```python
from build123d import *

# Parameters (mm, degrees)
F0_R     = 2.38125
F1_DEPTH = 2.54
F2_R     = 40.005
F2_R_2   = 28.575
F2_R_3   = 2.38125
F3_DEPTH = 2.5410001


with BuildPart() as f1:
    # F0 (on Front) → F1 (new body)
    with BuildSketch(Plane.XZ):
        with BuildLine():
            ThreePointArc((6.3499999233, -24.9008008357), (-1.0762466814, -6.9535395158), (-19.0125346344, 0.4991715332))
            ThreePointArc((-19.0125346344, 0.4991715332), (-154.4493523287, -0.8097271588), (-289.8234049708, -5.1353108434))
            add(Edge.make_bspline(
                [(-289.8234049708, -5.1353108434), (-514.6487503932, -20.2006873557), (-514.3499970436, -90.5002)],
                knots=[4.9283667006, 4.9283667006, 4.9283667006, 6.2844832596, 6.2844832596, 6.2844832596], degree=2, weights=[1, 0.7787921925, 1]))
            Line((-514.3499970436, -90.5002), (-514.3499970436, -249.2502))
            ThreePointArc((-514.3499970436, -249.2502), (-506.9105092857, -267.2107122421), (-488.9499970436, -274.6502))
            Line((-488.9499970436, -274.6502), (-373.0752, -274.6502))
            ThreePointArc((-373.0752, -274.6502), (-337.1541755157, -259.7712244843), (-322.2752, -223.8502))
            Line((-322.2752, -223.8502), (-322.2752, -211.0369156084))
            ThreePointArc((-322.2752, -211.0369156084), (-303.2252, -191.9869156084), (-284.1752, -211.0369156084))
            Line((-284.1752, -211.0369156084), (-284.1752, -223.7369156084))
            ThreePointArc((-284.1752, -223.7369156084), (-269.2962244843, -259.6579400927), (-233.3752, -274.5369156084))
            Line((-233.3752, -274.5369156084), (-19.0500000767, -274.5369156084))
            ThreePointArc((-19.0500000767, -274.5369156084), (-1.0894878346, -267.0974278505), (6.3499999233, -249.1369156084))
            Line((6.3499999233, -249.1369156084), (6.3499999233, -24.9008008357))
        make_face()
        with Locations((-412.75, -261.9502)):
            Circle(F0_R, mode=Mode.SUBTRACT)
        with Locations((-180.975, -261.9502)):
            Circle(F0_R, mode=Mode.SUBTRACT)
        with Locations((-34.925, -261.9502)):
            Circle(F0_R, mode=Mode.SUBTRACT)
        with BuildLine():
            ThreePointArc((-177.8000000767, -147.5369156084), (-175.9401281373, -143.0467875478), (-171.4500000767, -141.1869156084))
            Line((-171.4500000767, -141.1869156084), (-25.4000000767, -141.1869156084))
            ThreePointArc((-25.4000000767, -141.1869156084), (-20.9098720162, -143.0467875478), (-19.0500000767, -147.5369156084))
            Line((-19.0500000767, -147.5369156084), (-19.0500000767, -242.7869156084))
            ThreePointArc((-19.0500000767, -242.7869156084), (-20.9098720162, -247.2770436689), (-25.4000000767, -249.1369156084))
            Line((-25.4000000767, -249.1369156084), (-171.4500000767, -249.1369156084))
            ThreePointArc((-171.4500000767, -249.1369156084), (-175.9401281373, -247.2770436689), (-177.8000000767, -242.7869156084))
            Line((-177.8000000767, -242.7869156084), (-177.8000000767, -203.9237609675))
            ThreePointArc((-177.8000000767, -203.9237609675), (-180.3400000767, -196.9399156084), (-177.8000000767, -189.9560702493))
            Line((-177.8000000767, -189.9560702493), (-177.8000000767, -147.5369156084))
        make_face(mode=Mode.SUBTRACT)
        with Locations((-438.15, -46.0502)):
            Circle(F0_R, mode=Mode.SUBTRACT)
        with Locations((-228.6, -14.1869156084)):
            Circle(F0_R, mode=Mode.SUBTRACT)
        with Locations((-19.05, -11.1252)):
            Circle(F0_R, mode=Mode.SUBTRACT)
    extrude(amount=F1_DEPTH)

    # F2 (on face) → F3 (cut, through all)
    with BuildSketch(Plane.XZ.offset(2.54)):
        with Locations((-50.8, -93.5619156084)):
            Circle(F2_R)
        with Locations((-139.7, -93.5619156084)):
            Circle(F2_R)
        with Locations((-228.6, -93.5619156084)):
            Circle(F2_R)
        with Locations((-304.8, -118.9619156084)):
            Circle(F2_R_2)
        with Locations((-19.05, -125.3119156084)):
            Circle(F2_R_3)
        with Locations((-82.5499999959, -125.3119156124)):
            Circle(F2_R_3)
        with Locations((-82.5500000081, -61.8119156165)):
            Circle(F2_R_3)
        with Locations((-19.0500000122, -61.8119155962)):
            Circle(F2_R_3)
        with Locations((-280.9748, -142.7871156084)):
            Circle(F2_R_3)
        with Locations((-280.9748, -95.1367156084)):
            Circle(F2_R_3)
        with Locations((-328.6252, -95.1367156084)):
            Circle(F2_R_3)
        with Locations((-328.6252, -142.7871156084)):
            Circle(F2_R_3)
        with Locations((-228.6, -207.8619156084)):
            Circle(F2_R)
        with Locations((-387.35, -118.9619156084)):
            Circle(F2_R)
        with Locations((-387.35, -207.8619156084)):
            Circle(F2_R)
        with Locations((-171.4499999959, -125.3119156124)):
            Circle(F2_R_3)
        with Locations((-107.95, -125.3119156084)):
            Circle(F2_R_3)
        with Locations((-107.9500000122, -61.8119155962)):
            Circle(F2_R_3)
        with Locations((-171.4500000081, -61.8119156165)):
            Circle(F2_R_3)
        with Locations((-260.3499999959, -125.3119156124)):
            Circle(F2_R_3)
        with Locations((-196.85, -125.3119156084)):
            Circle(F2_R_3)
        with Locations((-196.8500000122, -61.8119155962)):
            Circle(F2_R_3)
        with Locations((-260.3500000081, -61.8119156165)):
            Circle(F2_R_3)
        with Locations((-260.3500000081, -176.1119156165)):
            Circle(F2_R_3)
        with Locations((-260.3499999959, -239.6119156124)):
            Circle(F2_R_3)
        with Locations((-196.8500000122, -176.1119155962)):
            Circle(F2_R_3)
        with Locations((-196.85, -239.6119156084)):
            Circle(F2_R_3)
        with Locations((-419.1000000081, -176.1119156165)):
            Circle(F2_R_3)
        with Locations((-355.6000000122, -176.1119155962)):
            Circle(F2_R_3)
        with Locations((-355.6, -239.6119156084)):
            Circle(F2_R_3)
        with Locations((-419.0999999959, -239.6119156124)):
            Circle(F2_R_3)
        with Locations((-355.6, -150.7119156084)):
            Circle(F2_R_3)
        with Locations((-419.1000000081, -87.2119156165)):
            Circle(F2_R_3)
        with Locations((-355.6000000122, -87.2119155962)):
            Circle(F2_R_3)
        with Locations((-419.0999999959, -150.7119156124)):
            Circle(F2_R_3)
    extrude(amount=-F3_DEPTH, mode=Mode.SUBTRACT)


solid = f1.part
```
Verification items for the finished model (mm, model axes). A direction names the side the tool comes from. Round coordinates to 2 decimals unless told otherwise and drop trailing zeros. Order: outer loops, then holes, each group sorted by start corner. A loop starts at its lowest first (then second) coordinate and runs counter-clockwise, first axis right, second up. Notation, with made-up numbers: (16, 65.5) - (22, 65.5) arc R23 cw to (22, 96.5) - close; hole circle Ø7 at (23, 85.25). An arc over 180 degrees is marked (long way). Use CSV: the item, a comma, the result in double quotes. Start each with the question number.
1) Access from +Z, -Z, +X, -X, +Y, -Y to the whole of each face (thin tool, end or side, straight path). Record for faces 1 (the cylindrical face through (-59.472, -1.288, -132.616)), 2 (the cylindrical face through (-337.55, -1.25, -260.16)).
2) Go/stop test with a flat-tipped pin: P1, Ø1.3, axis at x = -137, y = -1, coming from the -Z side. Record where the tip stops, or that it passes through.
3) Section check A-A, the plane x = -138.5. Record the cut outline in (y, z), plus the area to 3 significant figures.
4) Section check B-B, the plane y = -0.8. State how many separate pieces and enclosed holes the cut face has, plus the area to 3 significant figures.
5) Thickness scan on L1, parallel to Z at x = -52, y = -2.25; L2, parallel to Z at x = -405.5, y = -1; L3, parallel to X at y = -1.05, z = -82.5. Record the ranges inside material, lowest first.
Answers:
1,face 1,"+Y, -Y"
1,face 2,"-Z, +Y, -Y"
2,P1,"stops at z = -274.54"
3,outline,"(-2.54, -274.54) - (0, -274.54) - (0, -249.14) - (-2.54, -249.14) - close; (-2.54, -141.19) - (0, -141.19) - (0, -133.55) - (-2.54, -133.55) - close; (-2.54, -53.57) - (0, -53.57) - (0, -0.5) - (-2.54, -0.5) - close"
3,area,"219 mm²"
4,separate pieces,"1"
4,enclosed holes,"42"
4,area,"81,600 mm²"
5,L1,"z = -274.54 to -249.14, -141.19 to -133.55, -53.57 to 0.46"
5,L2,"z = -274.65 to -243.51, -172.21 to -154.61, -83.31 to -21.85"
5,L3,"x = -513.18 to -403.81, -370.89 to -267.05, -190.15 to -178.15, -101.25 to -89.25, -12.35 to 6.35"
